```python
from build123d import *

# Parameters (mm, degrees)
SKETCH1_W                      = 152.4
SKETCH1_H                      = 76.2
BOSS_EXTRUDE1_DEPTH            = 28.575
SKETCH2_R                      = 9.525
CUT_EXTRUDE1_DEPTH             = 13.462
CUT_EXTRUDE3_DEPTH             = 3.302
CUT_EXTRUDE4_DEPTH             = 7.62
F_7_0_201_DIAMETER_HOLE1_D     = 5.1054
F_7_0_201_DIAMETER_HOLE1_DEPTH = 14.2748
F_7_0_201_DIAMETER_HOLE1_TIP   = 1.533816902
SKETCH10_OUTSIDE_W             = 188.954
SKETCH10_OUTSIDE_H             = 112.754
CUT_EXTRUDE5_DEPTH             = 12.7
CIRPATTERN1_COUNT              = 6


with BuildPart() as part:
    # Sketch1 → Boss-Extrude1 (new body)
    with BuildSketch(Plane(origin=(0, 0, 0), x_dir=(1, 0, 0), z_dir=(0, 1, 0))):
        Rectangle(SKETCH1_W, SKETCH1_H)
    extrude(amount=BOSS_EXTRUDE1_DEPTH)

    # Sketch2 → Cut-Extrude1 (cut)
    with BuildSketch(Plane(origin=(0, 28.575, 0), x_dir=(1, 0, 0), z_dir=(0, 1, 0))):
        Circle(SKETCH2_R)
    extrude(amount=-CUT_EXTRUDE1_DEPTH, mode=Mode.SUBTRACT)

    # Sketch4 → Cut-Extrude3 (cut)
    with BuildSketch(Plane(origin=(0, 28.575, 0), x_dir=(1, 0, 0), z_dir=(0, 1, 0))):
        with BuildLine():
            Line((-36.2712, 33.3375), (37.288597325, 33.3375))
            ThreePointArc((37.288597325, 33.3375), (48.293963964, 28.161232705), (51.324986679, 16.383086023))
            Line((51.324986679, 16.383086023), (42.614045782, -29.463971326))
            ThreePointArc((42.614045782, -29.463971326), (40.9723269, -32.243455546), (37.935249331, -33.3375))
            Line((37.935249331, -33.3375), (-42.6212, -33.3375))
            ThreePointArc((-42.6212, -33.3375), (-45.988796045, -31.942596045), (-47.3837, -28.575))
            Line((-47.3837, -28.575), (-47.3837, 22.225))
            ThreePointArc((-47.3837, 22.225), (-44.128924106, 30.082724106), (-36.2712, 33.3375))
        make_face()
        with BuildLine():
            ThreePointArc((-36.2712, 30.1625), (-41.883860076, 27.837660076), (-44.2087, 22.225))
            Line((-44.2087, 22.225), (-44.2087, -28.575))
            ThreePointArc((-44.2087, -28.575), (-43.743732015, -29.697532015), (-42.6212, -30.1625))
            Line((-42.6212, -30.1625), (37.935249331, -30.1625))
            ThreePointArc((37.935249331, -30.1625), (38.947608521, -29.797818515), (39.494848148, -28.871323775))
            Line((39.494848148, -28.871323775), (48.205789045, 16.975733573))
            ThreePointArc((48.205789045, 16.975733573), (45.848326933, 26.136514326), (37.288597325, 30.1625))
            Line((37.288597325, 30.1625), (-36.2712, 30.1625))
        make_face(mode=Mode.SUBTRACT)
    extrude(amount=-CUT_EXTRUDE3_DEPTH, mode=Mode.SUBTRACT)

    # Sketch7 → Cut-Extrude4 (cut)
    with BuildSketch(Plane(origin=(0, 28.575, 0), x_dir=(1, 0, 0), z_dir=(0, 1, 0))):
        with BuildLine():
            Line((31.75, 20.6375), (31.75, -20.6375))
            ThreePointArc((31.75, -20.6375), (30.355096045, -24.005096045), (26.9875, -25.4))
            Line((26.9875, -25.4), (-26.9875, -25.4))
            ThreePointArc((-26.9875, -25.4), (-30.355096045, -24.005096045), (-31.75, -20.6375))
            Line((-31.75, -20.6375), (-31.75, 20.6375))
            ThreePointArc((-31.75, 20.6375), (-30.355096045, 24.005096045), (-26.9875, 25.4))
            Line((-26.9875, 25.4), (26.9875, 25.4))
            ThreePointArc((26.9875, 25.4), (30.355096045, 24.005096045), (31.75, 20.6375))
        make_face()
    extrude(amount=-CUT_EXTRUDE4_DEPTH, mode=Mode.SUBTRACT)

    # #7 (0.201) Diameter Hole1
    with Locations(Plane(origin=(0, 28.575, 0), x_dir=(-1, 0, 0), z_dir=(0, 1, 0))):
        with Locations((66.675, -28.575), (-66.675, -28.575), (-66.675, 28.575), (66.675, 28.575)):
            Hole(F_7_0_201_DIAMETER_HOLE1_D / 2, depth=F_7_0_201_DIAMETER_HOLE1_DEPTH)
            with Locations((0, 0, -(F_7_0_201_DIAMETER_HOLE1_DEPTH + F_7_0_201_DIAMETER_HOLE1_TIP / 2))):  # 118° drill point
                Cone(0, F_7_0_201_DIAMETER_HOLE1_D / 2, F_7_0_201_DIAMETER_HOLE1_TIP, mode=Mode.SUBTRACT)

    # Sketch10 outside → Cut-Extrude5 (cut)
    with BuildSketch(Plane(origin=(0, 28.575, 0), x_dir=(1, 0, 0), z_dir=(0, 1, 0))):
        Rectangle(SKETCH10_OUTSIDE_W, SKETCH10_OUTSIDE_H)
        with BuildLine():
            Line((-73.025, 32.54502), (-73.025, -32.54502))
            ThreePointArc((-73.025, -32.54502), (-72.09506403, -34.79008403), (-69.85, -35.72002))
            Line((-69.85, -35.72002), (69.85, -35.72002))
            ThreePointArc((69.85, -35.72002), (72.09506403, -34.79008403), (73.025, -32.54502))
            Line((73.025, -32.54502), (73.025, 32.54502))
            ThreePointArc((73.025, 32.54502), (72.09506403, 34.79008403), (69.85, 35.72002))
            Line((69.85, 35.72002), (-69.85, 35.72002))
            ThreePointArc((-69.85, 35.72002), (-72.09506403, 34.79008403), (-73.025, 32.54502))
        make_face(mode=Mode.SUBTRACT)
    extrude(amount=-CUT_EXTRUDE5_DEPTH, mode=Mode.SUBTRACT)

    # Sketch13 → 1/8 (0.125) Diameter Hole1 (revolve, cut)
    with BuildSketch(Plane(origin=(14.964433671, 20.955, -5.29918389), x_dir=(0, 0, 1), z_dir=(1, 0, 0))):
        Polygon((0, 0), (0, 18.429066233), (1.5875, 17.4752), (1.5875, 0), align=None)
    f_1_8_0_125_diameter_hole1 = revolve(axis=Axis((14.964433671, 27.305, -5.29918389), (0, -1, 0)), mode=Mode.SUBTRACT)

    # CirPattern1: 1/8 (0.125) Diameter Hole1 ×6 about axis
    cirpattern1_axis = Axis((0, 0, 0), (0, 1, 0))
    for i in range(1, CIRPATTERN1_COUNT):
        add(f_1_8_0_125_diameter_hole1.rotate(cirpattern1_axis, i * 360 / CIRPATTERN1_COUNT), mode=Mode.SUBTRACT)


solid = part.part
```
Work out the finished part from the listing and answer in its coordinate system (mm). A direction names the side the tool comes from. Give positions to 0.01 mm unless a question says otherwise; leave off trailing zeros. Loops run counter-clockwise (first coordinate to the right, second up) from the corner with the lowest first, then second, coordinate; pieces in that order, holes last. Notation, with made-up numbers: (3.5, 7.25) -> (33.5, 7.25) arc R12 ccw to (33.5, 12.25) -> close; hole circle Ø9 at (-18.5, -11). An arc over 180 degrees is marked (long way). Write item = value, one per line. Start each with the question number.
(1) Find section A-A on x = 19.5. Give the vertices of the cut face in (y, z) (1 decimal), and give its area (3 significant figures).
(2) The mould has two halves that part along X. Classify faces 1 (the flat face through (73.025, 22, 0)), 2 (the cylindrical face through (45.935, 26.947, -26.031)), 3 (the flat face through (1, 22, -35.72)), 4 (the flat face through (-76.2, 8, 1)): +X half, -X half, draft (parallel to the pull), parting line (faces both ways), or undercut.
(3) Find the intervals of material crossed by probe 1 along X at (y, z) = (3.75, 10.5); probe 2 along X at (y, z) = (21.25, -21) (3 decimals); probe 3 along Z at (x, y) = (-3, 18.5), in increasing order. Write a range as from..to.
(4) Which of the six approach directions +Z, -Z, +X, -X, +Y, -Y give full straight-line access (tool end or side, diameter ignored) to faces 5 (the flat face through (0, 15.113, 0)), 6 (the cylindrical face through (72.12, 22.314, -34.765)), 7 (the flat face through (76.2, 8, 1))?
(5) Find section C-C on x = 59.5. Give the vertices of the cut face in (y, z) (3 decimals), and give its area (3 significant figures).
(6) Given pin 1 Ø6.5 at (y, z) = (23.5, 13) entering from -X (3 decimals); pin 2 Ø2.5 at (x, z) = (-14.96, 5.3) entering from +Y; pin 3 Ø5.5 at (x, z) = (0.5, 4) entering from +Y, each flat-ended and moving along its own axis, determine where each tip first touches the part or whether it passes through.
(7) Find section B-B on z = 0. Give the vertices of the cut face in (x, y) (3 decimals), and give its area (3 significant figures).
From the geometry:
q1.outline = (0, -38.1) -> (15.9, -38.1) -> (15.9, -35.7) -> (28.6, -35.7) -> (28.6, -33.3) -> (25.3, -33.3) -> (25.3, -30.2) -> (28.6, -30.2) -> (28.6, -25.4) -> (21, -25.4) -> (21, 25.4) -> (28.6, 25.4) -> (28.6, 30.2) -> (25.3, 30.2) -> (25.3, 33.3) -> (28.6, 33.3) -> (28.6, 35.7) -> (15.9, 35.7) -> (15.9, 38.1) -> (0, 38.1) -> close
q1.area = 1,710 mm^2
q2.face_1 = +X half
q2.face_2 = undercut
q2.face_3 = draft
q2.face_4 = -X half
q3.probe_1 = -76.2..10.5, 13.65..76.2
q3.probe_2 = -73.025..-31.736, 31.736..73.025
q3.probe_3 = -35.72..-9.04, 9.04..14.03, 17.19..35.72
q4.face_5 = +Y
q4.face_6 = -Z, +X, +Y
q4.face_7 = +Z, -Z, +X, +Y, -Y
q5.outline = (0, -38.1) -> (15.875, -38.1) -> (15.875, -35.72) -> (28.575, -35.72) -> (28.575, 35.72) -> (15.875, 35.72) -> (15.875, 38.1) -> (0, 38.1) -> close
q5.area = 2,120 mm^2
q6.pin_1 = -73.025
q6.pin_2 = 3.28
q6.pin_3 = 15.11
q7.outline = (-76.2, 0) -> (76.2, 0) -> (76.2, 15.875) -> (73.025, 15.875) -> (73.025, 28.575) -> (48.212, 28.575) -> (48.212, 25.273) -> (44.98, 25.273) -> (44.98, 28.575) -> (31.75, 28.575) -> (31.75, 20.955) -> (9.525, 20.955) -> (9.525, 15.113) -> (-9.525, 15.113) -> (-9.525, 20.955) -> (-31.75, 20.955) -> (-31.75, 28.575) -> (-44.209, 28.575) -> (-44.209, 25.273) -> (-47.384, 25.273) -> (-47.384, 28.575) -> (-73.025, 28.575) -> (-73.025, 15.875) -> (-76.2, 15.875) -> close
q7.area = 3,660 mm^2
